Print and shaded views of the part. All mm, measured from the part's lowest x, y and z. Coordinates: 2 decimals unless noted, no trailing zeros. Order: outer loops, then holes, each group sorted by start corner. A loop starts at its lowest first (then second) coordinate and runs counter-clockwise, first axis right, second up. Notation, with made-up numbers: (5, 72) -> (44, 72) arc R26 cw to (44, 91) -> close; hole circle Ø5 at (9, 50.25). An arc over 180 degrees is marked (long way). Return JSON: item names as keys, results as strings. Group by question number.
1) Cut at D-D (z = 1.45). Write the cut outline in (x, y), and give its area (3 significant figures).
2) Cut at B-B (x = 12.5). Write the cut outline in (y, z), and give its area (3 significant figures).
3) Cut at A-A (y = 45). Write the cut outline in (x, z).
4) Cut at C-C (y = 12.5). Write the cut outline in (x, z).
5) Probe line 1 (Y direction, x = 157.5, z = 1.85); line 2 (Y direction, x = 85, z = 1.15); line 3 (X direction, y = 14.5, z = 2.05). List the from-to ranges inside material, lowest first.
6) Flat gauge pin, fed straight in: pin 1 (3 mm diameter, centred on x = 12.5, y = 12.5, fed in from +Z). Where does the tip first touch, or does it go through?
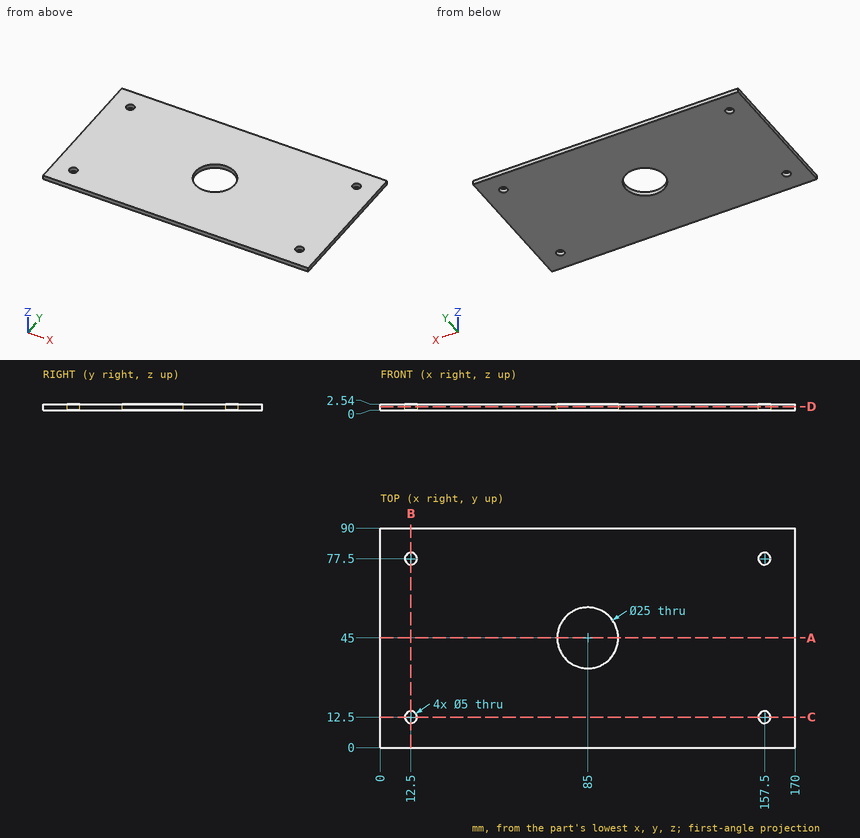
Answers below:
{
 "1": {"outline": "(0, 0) -> (170, 0) -> (170, 90) -> (0, 90) -> close; hole circle Ø5 at (12.5, 12.5); hole circle Ø5 at (12.5, 77.5); hole circle Ø25 at (85, 45); hole circle Ø5 at (157.5, 12.5); hole circle Ø5 at (157.5, 77.5)", "area": "14,700 mm^2"},
 "2": {"outline": "(0, 0) -> (10, 0) -> (10, 2.54) -> (0, 2.54) -> close; (15, 0) -> (75, 0) -> (75, 2.54) -> (15, 2.54) -> close; (80, 0) -> (90, 0) -> (90, 2.54) -> (80, 2.54) -> close", "area": "203 mm^2"},
 "3": {"outline": "(0, 0) -> (72.5, 0) -> (72.5, 2.54) -> (0, 2.54) -> close; (97.5, 0) -> (170, 0) -> (170, 2.54) -> (97.5, 2.54) -> close"},
 "4": {"outline": "(0, 0) -> (10, 0) -> (10, 2.54) -> (0, 2.54) -> close; (15, 0) -> (155, 0) -> (155, 2.54) -> (15, 2.54) -> close; (160, 0) -> (170, 0) -> (170, 2.54) -> (160, 2.54) -> close"},
 "5": {"line 1": "y = 0 to 10, 15 to 75, 80 to 90", "line 2": "y = 0 to 32.5, 57.5 to 90", "line 3": "x = 0 to 11, 14 to 156, 159 to 170"},
 "6": {"pin 1": "passes through"}
}
